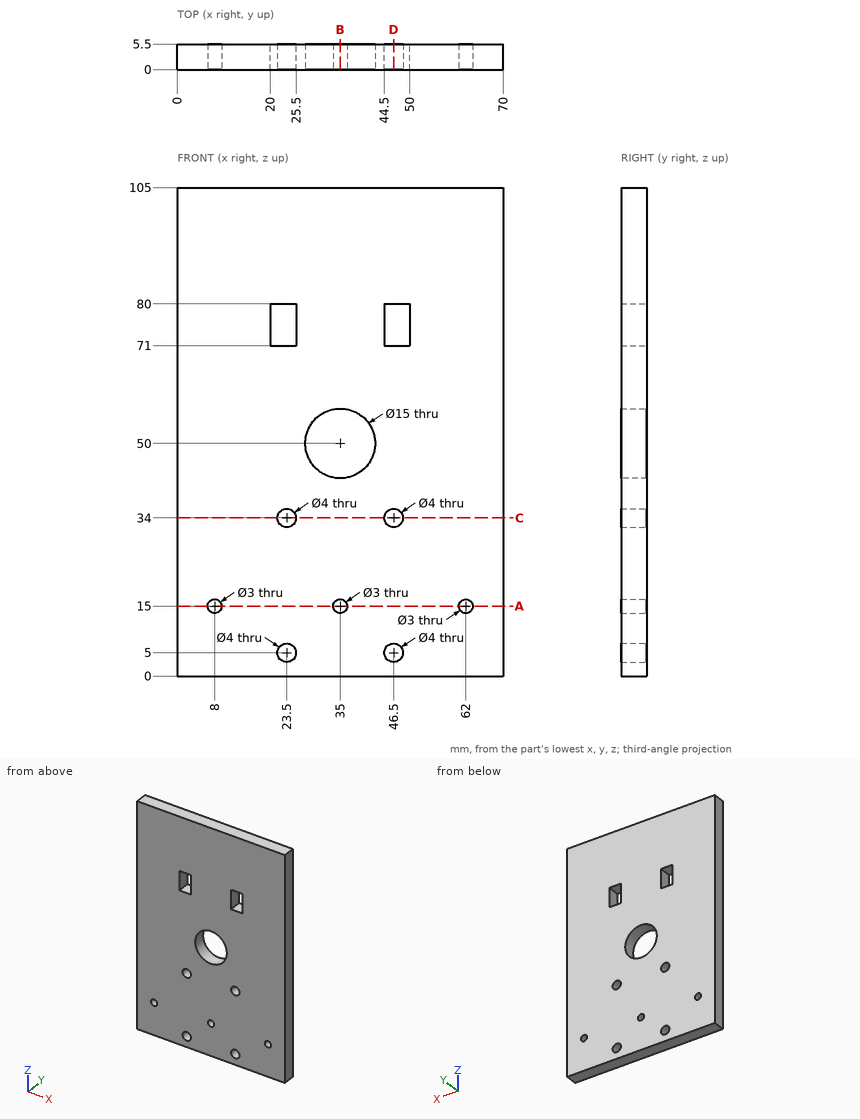
The drawing under review shows one solid part. Ordinate dimensions are in mm from its lowest x, y, z. Coordinates: 2 decimals unless noted, no trailing zeros. Order: outer loops, then holes, each group sorted by start corner. A loop starts at its lowest first (then second) coordinate and runs counter-clockwise, first axis right, second up. Notation, with made-up numbers: (13.5, 62.25) -> (59.5, 62.25) arc R22 ccw to (59.5, 86.25) -> close; hole circle Ø6 at (-7, 24.25). An arc over 180 degrees is marked (long way). Answer in a Markdown table with one row per item. Add a question column.
Item 1: To check wall thickness, follow probe 1 along X at (y, z) = (3.8, 5); probe 2 along X at (y, z) = (0.3, 71.5); probe 3 along X at (y, z) = (1.1, 15). State the ranges of each line that lie inside material, in increasing order.
Item 2: We need section B-B on x = 35. Write out the cut boundary in (y, z), plus the area to 4 significant figures.
Item 3: We need section C-C on z = 34. Write out the cut boundary in (x, y).
Item 4: We need section D-D on x = 46.5. Write out the cut boundary in (y, z), plus the area to 3 significant figures.
Item 5: We need section A-A on z = 15. Write out the cut boundary in (x, y).
Final values:
| question | item | result |
|---|---|---|
| 1 | probe 1 | x = 0 to 21.5, 25.5 to 44.5, 48.5 to 70 |
| 1 | probe 2 | x = 0 to 20, 25.5 to 44.5, 50 to 70 |
| 1 | probe 3 | x = 0 to 6.5, 9.5 to 33.5, 36.5 to 60.5, 63.5 to 70 |
| 2 | outline | (0, 0) -> (5.5, 0) -> (5.5, 13.5) -> (0, 13.5) -> close; (0, 16.5) -> (5.5, 16.5) -> (5.5, 42.5) -> (0, 42.5) -> close; (0, 57.5) -> (5.5, 57.5) -> (5.5, 105) -> (0, 105) -> close |
| 2 | area | 478.5 mm2 |
| 3 | outline | (0, 0) -> (21.5, 0) -> (21.5, 5.5) -> (0, 5.5) -> close; (25.5, 0) -> (44.5, 0) -> (44.5, 5.5) -> (25.5, 5.5) -> close; (48.5, 0) -> (70, 0) -> (70, 5.5) -> (48.5, 5.5) -> close |
| 4 | outline | (0, 0) -> (5.5, 0) -> (5.5, 3) -> (0, 3) -> close; (0, 7) -> (5.5, 7) -> (5.5, 32) -> (0, 32) -> close; (0, 36) -> (5.5, 36) -> (5.5, 71) -> (0, 71) -> close; (0, 80) -> (5.5, 80) -> (5.5, 105) -> (0, 105) -> close |
| 4 | area | 484 mm2 |
| 5 | outline | (0, 0) -> (6.5, 0) -> (6.5, 5.5) -> (0, 5.5) -> close; (9.5, 0) -> (33.5, 0) -> (33.5, 5.5) -> (9.5, 5.5) -> close; (36.5, 0) -> (60.5, 0) -> (60.5, 5.5) -> (36.5, 5.5) -> close; (63.5, 0) -> (70, 0) -> (70, 5.5) -> (63.5, 5.5) -> close |
